```python
from build123d import *

# Parameters (mm, degrees)
F1_DEPTH = 1.5
F2_R     = 0.5
F4_DEPTH = 15


with BuildPart() as f1:
    # F0 (on Top) → F1 (new body, symmetric)
    with BuildSketch(Plane.XY):
        with BuildLine():
            ThreePointArc((-5, -2.5), (-4.8535533906, -2.8535533906), (-4.5, -3))
            Line((-4.5, -3), (4.5, -3))
            ThreePointArc((4.5, -3), (4.8535533906, -2.8535533906), (5, -2.5))
            Line((5, -2.5), (5, 2.5))
            ThreePointArc((5, 2.5), (4.8535533906, 2.8535533906), (4.5, 3))
            Line((4.5, 3), (-4.5, 3))
            ThreePointArc((-4.5, 3), (-4.8535533906, 2.8535533906), (-5, 2.5))
            Line((-5, 2.5), (-5, -2.5))
        make_face()
    extrude(amount=F1_DEPTH, both=True)

    # F2
    f2_edges = [f1.edges().sort_by_distance(p)[0] for p in [
        (0, 3, 1.5),
        (-5, 0, -1.5),
    ]]
    fillet(f2_edges, radius=F2_R)

    # F3 (on Right) → F4 (cut, symmetric)
    with BuildSketch(Plane.YZ):
        with BuildLine():
            ThreePointArc((0, -0.0614410286), (0.0037479373, -0.03082207), (0.005, 0))
            ThreePointArc((0.005, 0), (0.0037479373, 0.03082207), (0, 0.0614410286))
            ThreePointArc((0, 0.0614410286), (-0.005, 0), (0, -0.0614410286))
        make_face()
        with BuildLine():
            ThreePointArc((0, 0.0614410286), (0.0037479373, 0.03082207), (0.005, 0))
            ThreePointArc((0.005, 0), (0.0037479373, -0.03082207), (0, -0.0614410286))
            ThreePointArc((0, -0.0614410286), (0.40582207, -0.3787479373), (0.755, 0))
            ThreePointArc((0.755, 0), (0.40582207, 0.3787479373), (0, 0.0614410286))
        make_face()
        with BuildLine():
            ThreePointArc((0, -0.0614410286), (-0.005, 0), (0, 0.0614410286))
            ThreePointArc((0, 0.0614410286), (-0.755, 0), (0, -0.0614410286))
        make_face()
    extrude(amount=F4_DEPTH, both=True, mode=Mode.SUBTRACT)


solid = f1.part
```
Input: part model. Units: mm. Frame: model coordinates. Round coordinates to 2 decimals unless told otherwise and drop trailing zeros. Order: outer loops, then holes, each group sorted by start corner. A loop starts at its lowest first (then second) coordinate and runs counter-clockwise, first axis right, second up. Notation, with made-up numbers: (31, 22.25) - (90, 22.25) arc R26 cw to (90, 42.25) - close; hole circle Ø7 at (84.5, 74.5). An arc over 180 degrees is marked (long way). Answer in a Markdown table with one row per item.
Item 1: Section query C-C (x = -0.5). Return the cut outline in (y, z) (3 decimals).
Model answer:
| item | result |
|---|---|
| outline | (-3, -1) arc R0.5 ccw to (-2.5, -1.5) - (2.5, -1.5) arc R0.5 ccw to (3, -1) - (3, 1) arc R0.5 ccw to (2.5, 1.5) - (-2.5, 1.5) arc R0.5 ccw to (-3, 1) - close; hole (0, -0.061) arc R0.38 ccw (long way) to (0, 0.061) arc R0.38 ccw (long way) to start |
Item 2: Line query: line 1 (Y direction, x = -1.75, z = 0) (3 decimals); line 2 (X direction, y = -1.5, z = -1.05); line 3 (Z direction, x = -3, y = -0.5). Output: solid intervals per line, ascending.
Model answer:
| item | result |
|---|---|
| line 1 | y = -3 to -0.755, 0.755 to 3 |
| line 2 | x = -5 to 5 |
| line 3 | z = -1.5 to -0.36, 0.36 to 1.5 |
Item 3: Section query B-B (z = 0.2). Return the cut outline in (x, y), then the cut area to 3 significant figures.
Model answer:
| item | result |
|---|---|
| outline | (-5, -2.5) arc R0.5 ccw to (-4.5, -3) - (4.5, -3) arc R0.5 ccw to (5, -2.5) - (5, -0.7) - (-5, -0.7) - close; (-5, -0.05) - (5, -0.05) - (5, 0.05) - (-5, 0.05) - close; (-5, 0.7) - (5, 0.7) - (5, 2.5) arc R0.5 ccw to (4.5, 3) - (-4.5, 3) arc R0.5 ccw to (-5, 2.5) - close |
| area | 46.9 mm² |
Item 4: Section query A-A (y = -0.25). Return the cut outline in (x, z), then the cut area to 3 significant figures.
Model answer:
| item | result |
|---|---|
| outline | (-5, -1) arc R0.5 ccw to (-4.5, -1.5) - (4.5, -1.5) arc R0.5 ccw to (5, -1) - (5, -0.36) - (-5, -0.36) - close; (-5, 0.36) - (5, 0.36) - (5, 1) arc R0.5 ccw to (4.5, 1.5) - (-4.5, 1.5) arc R0.5 ccw to (-5, 1) - close |
| area | 22.6 mm² |
